Geometry check sheet. Reference: the model listing, model coordinates, mm. A direction names the side the tool comes from. Give positions to 0.01 mm unless a question says otherwise; leave off trailing zeros. Loops run counter-clockwise (first coordinate to the right, second up) from the corner with the lowest first, then second, coordinate; pieces in that order, holes last. Notation, with made-up numbers: (-1.75, 76.5) -> (40.25, 76.5) arc R6 ccw to (40.25, 80.5) -> close; hole circle Ø10 at (-22, 87). An arc over 180 degrees is marked (long way). Write item = value, one per line. Start each with the question number.
```python
from build123d import *

# Parameters (mm, degrees)
EXTRUDE_1_DEPTH     = 3
SKETCH_2_R          = 1.35
CUT_EXTRUDE_1_DEPTH = 124.729543764
SKETCH_3_R          = 1.1
CUT_EXTRUDE_2_DEPTH = 124.729543764
EXTRUDE_2_DEPTH     = 3
FILLET_1_R          = 10
FILLET_2_R          = 2


with BuildPart() as part:
    # 草图1 → 凸台-拉伸1 (new body)
    with BuildSketch(Plane(origin=(0, 0, 0), x_dir=(1, 0, 0), z_dir=(0, 1, 0))):
        Polygon((10, 10), (10, 30), (-10, 30), (-10, -30), (10, -30), (10, -10), (120, -10), (120, 10), (120, 30), (100, 30), (100, 10), align=None)
    extrude(amount=EXTRUDE_1_DEPTH)

    # 草图2 → 切除-拉伸1 (cut, through all)
    with BuildSketch(Plane(origin=(0, 3, 0), x_dir=(1, 0, 0), z_dir=(0, 1, 0))):
        with Locations(Location((-6, 26, 0), (0, 0, 270))):
            Circle(SKETCH_2_R)
        with Locations(Location((-6, 14, 0), (0, 0, 90))):
            Circle(SKETCH_2_R)
        with Locations(Location((6, 14, 0), (0, 0, 270))):
            Circle(SKETCH_2_R)
        with Locations(Location((6, 26, 0), (0, 0, 90))):
            Circle(SKETCH_2_R)
        with Locations(Location((6, -26, 0), (0, 0, 270))):
            Circle(SKETCH_2_R)
        with Locations(Location((6, -14, 0), (0, 0, 90))):
            Circle(SKETCH_2_R)
        with Locations(Location((-6, -14, 0), (0, 0, 270))):
            Circle(SKETCH_2_R)
        with Locations(Location((-6, -26, 0), (0, 0, 90))):
            Circle(SKETCH_2_R)
        with Locations(Location((110, 6.5, 0), (0, 0, 270))):
            Circle(SKETCH_2_R)
        with Locations(Location((20, 6.5, 0), (0, 0, 90))):
            Circle(SKETCH_2_R)
        with Locations(Location((65, 6.5, 0), (0, 0, 270))):
            Circle(SKETCH_2_R)
        with Locations(Location((65, -6.5, 0), (0, 0, 90))):
            Circle(SKETCH_2_R)
        with Locations(Location((20, -6.5, 0), (0, 0, 270))):
            Circle(SKETCH_2_R)
        with Locations(Location((110, -6.5, 0), (0, 0, 90))):
            Circle(SKETCH_2_R)
        with Locations(Location((104, 26, 0), (0, 0, 270))):
            Circle(SKETCH_2_R)
        with Locations(Location((104, 14, 0), (0, 0, 90))):
            Circle(SKETCH_2_R)
        with Locations(Location((116, 14, 0), (0, 0, 270))):
            Circle(SKETCH_2_R)
        with Locations(Location((116, 26, 0), (0, 0, 90))):
            Circle(SKETCH_2_R)
    extrude(amount=-CUT_EXTRUDE_1_DEPTH, mode=Mode.SUBTRACT)

    # 草图3 → 切除-拉伸2 (cut, through all)
    with BuildSketch(Plane(origin=(0, 3, 0), x_dir=(1, 0, 0), z_dir=(0, 1, 0))):
        with Locations(Location((115, 0, 0), (0, 0, 270))):
            Circle(SKETCH_3_R)
        with Locations(Location((100, 0, 0), (0, 0, 270))):
            Circle(SKETCH_3_R)
        with Locations(Location((85, 0, 0), (0, 0, 270))):
            Circle(SKETCH_3_R)
        with Locations(Location((70, 0, 0), (0, 0, 270))):
            Circle(SKETCH_3_R)
        with Locations(Location((55, 0, 0), (0, 0, 270))):
            Circle(SKETCH_3_R)
        with Locations(Location((40, 0, 0), (0, 0, 270))):
            Circle(SKETCH_3_R)
        with Locations(Location((25, 0, 0), (0, 0, 270))):
            Circle(SKETCH_3_R)
        with Locations(Location((10, 0, 0), (0, 0, 270))):
            Circle(SKETCH_3_R)
        with Locations(Location((-5, 0, 0), (0, 0, 270))):
            Circle(SKETCH_3_R)
    extrude(amount=-CUT_EXTRUDE_2_DEPTH, mode=Mode.SUBTRACT)

    # 草图4 → 凸台-拉伸2 (add)
    with BuildSketch(Plane(origin=(0, 3, 0), x_dir=(1, 0, 0), z_dir=(0, 1, 0))):
        Polygon((10, -30), (20, -10), (10, -10), align=None)
        Polygon((20, 10), (10, 10), (10, 30), align=None)
        Polygon((100, 30), (90, 10), (100, 10), align=None)
    extrude(amount=-EXTRUDE_2_DEPTH)

    # 圆角1
    fillet_1_edges = [part.edges().sort_by_distance(p)[0] for p in [
        (20, 1.5, -10),
        (20, 1.5, 10),
        (90, 1.5, -10),
        (10, 1.5, -30),
        (100, 1.5, -30),
        (10, 1.5, 30),
    ]]
    fillet(fillet_1_edges, radius=FILLET_1_R)

    # 圆角2
    fillet_2_edges = [part.edges().sort_by_distance(p)[0] for p in [
        (120, 1.5, -30),
        (120, 1.5, 10),
        (-10, 1.5, 30),
        (-10, 1.5, -30),
    ]]
    fillet(fillet_2_edges, radius=FILLET_2_R)


solid = part.part
```
1) Section check D-D (x = 49). Enter the section's corners in (y, z), plus the area to 3 significant figures.
2) Section check C-C (y = 2.5). Give the number of separate pieces and of enclosed holes in the cut face, plus the area to 3 significant figures.
3) Section check A-A (x = 65). Enter the section's corners in (y, z), plus the area to 3 significant figures.
4) Draft check along X on faces 1 (the flat face through (120, 1, -10)), 2 (the flat face through (54, 0, -7)), 3 (the cylindrical face through (6.406, 1.521, 27.288)). Enter one of: released by +X, released by -X, zero draft, split by the parting line, or undercut.
5) Depth check by flat-ended pin: pin 1 Ø1.5 at (y, z) = (0.5, 14) entering from +X; pin 2 Ø1.5 at (y, z) = (1, 15.5) entering from +X. Enter the tip coordinate at first touch or a pass-through.
6) Tool access check on faces 4 (the cylindrical face through (104.406, 1.521, -24.712)), 5 (the flat face through (15, 2, -20)). Record the directions out of +Z, -Z, +X, -X, +Y, -Y that give a thin tool (end or side, any length) a straight path to the whole face; none if there is none.
7) Thickness scan on line 1 (X direction, y = 1.9, z = 6.5); line 2 (Z direction, x = 110, y = 0.95); line 3 (X direction, y = 1.85, z = -26). Record the ranges inside material, lowest first.
8) Section check B-B (z = 14). Enter the section's corners in (x, y), plus the area to 3 significant figures.
Check result:
q1.outline = (0, -10) -> (3, -10) -> (3, 10) -> (0, 10) -> close
q1.area = 60.0 mm2
q2.separate_pieces = 1
q2.enclosed_holes = 27
q2.area = 3,960 mm2
q3.outline = (0, -10) -> (3, -10) -> (3, -7.85) -> (0, -7.85) -> close; (0, -5.15) -> (3, -5.15) -> (3, 5.15) -> (0, 5.15) -> close; (0, 7.85) -> (3, 7.85) -> (3, 10) -> (0, 10) -> close
q3.area = 43.8 mm2
q4.face_1 = released by +X
q4.face_2 = zero draft
q4.face_3 = undercut
q5.pin_1 = 18.8
q5.pin_2 = 17.67
q6.face_4 = +Y, -Y
q6.face_5 = -Z, +Y, -Y
q7.line_1 = -10 to 18.65, 21.35 to 63.65, 66.35 to 108.65, 111.35 to 120
q7.line_2 = -30 to -7.85, -5.15 to 5.15, 7.85 to 10
q7.line_3 = -10 to -7.35, -4.65 to 4.65, 7.35 to 11.82, 98.18 to 102.65, 105.35 to 114.65, 117.35 to 120
q8.outline = (-10, 0) -> (-7.35, 0) -> (-7.35, 3) -> (-10, 3) -> close; (-4.65, 0) -> (4.65, 0) -> (4.65, 3) -> (-4.65, 3) -> close; (7.35, 0) -> (18.18, 0) -> (18.18, 3) -> (7.35, 3) -> close
q8.area = 68.3 mm2
